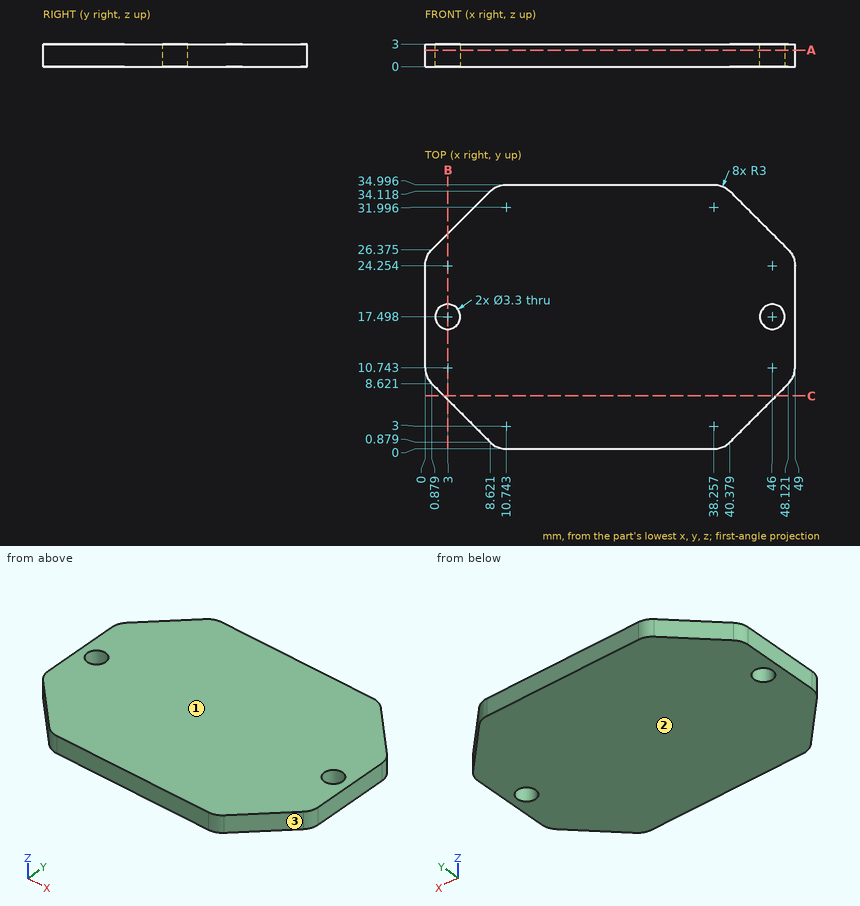
Check sheet for the drawn part. Datum: minimum x, y, z corner. Units: mm. Round coordinates to 2 decimals unless told otherwise and drop trailing zeros. Loops run counter-clockwise (first coordinate to the right, second up) from the corner with the lowest first, then second, coordinate; pieces in that order, holes last.
Item 1: Thickness scan on line 1 (X direction, y = 18, z = 0.15); line 2 (X direction, y = 24.5, z = 1.35); line 3 (X direction, y = 18.5, z = 1.9). Record the ranges inside material, lowest first.
Item 2: Mould release check, pull along Z, two halves, no side actions. Record for the marked faces 1, 2 and 3: pulls with the +Z half, pulls with the -Z half, needs draft (parallel to the pull), parting line crosses it, or undercut.
Item 3: Cross-section at C-C on y = 7. Record the boundary of the cut face in (x, z), then the cut area to 3 significant figures.
Item 4: Cross-section at A-A on z = 2.2. Count the separate pieces of the cut face and the enclosed holes in it, then the cut area to 3 significant figures.
Item 5: Cross-section at B-B on x = 3. Record the boundary of the cut face in (y, z).
Item 6: Gauge pin test, flat end, axial feed: pin 1 (1.5 mm diameter, centred on y = 31, z = 1.5, fed in from -X) (1 decimal). Record the tip position at first contact, or that the pin passes through.
Answer sheet:
1. line 1: x = 0 to 1.43, 4.57 to 44.43, 47.57 to 49
1. line 2: x = 0.01 to 48.99
1. line 3: x = 0 to 1.69, 4.31 to 44.69, 47.31 to 49
2. face 1: pulls with the +Z half
2. face 2: pulls with the -Z half
2. face 3: needs draft
3. outline: (2.5, 0) - (46.5, 0) - (46.5, 3) - (2.5, 3) - close
3. area: 132 mm2
4. separate pieces: 1
4. enclosed holes: 2
4. area: 1,520 mm2
5. outline: (6.5, 0) - (15.85, 0) - (15.85, 3) - (6.5, 3) - close; (19.15, 0) - (28.5, 0) - (28.5, 3) - (19.15, 3) - close
6. pin 1: stops at x = 4.8
